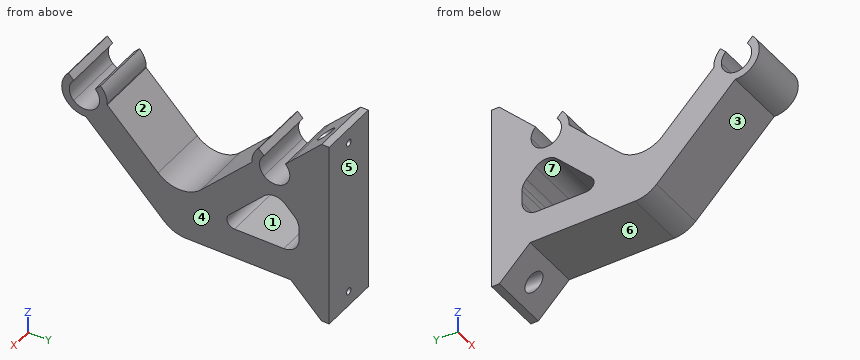
from build123d import *

# Parameters (mm, degrees)
F1_DEPTH = 50.8
F2_R     = 2.8575
F3_DEPTH = 224.1419342397
F5_R     = 6.35
F5_R_2   = 2.8575
F6_DEPTH = 217.7919342397


with BuildPart() as f1:
    # F0 (on Right) → F1 (new body)
    with BuildSketch(Plane.YZ):
        with BuildLine():
            Line((-66.2205500581, -66.2205500581), (-70.7106781187, -70.7106781187))
            ThreePointArc((-70.7106781187, -70.7106781187), (-65.8235712608, -75.2811893269), (-60.6417499855, -79.5146411593))
            ThreePointArc((-60.6417499855, -79.5146411593), (-62.1249501408, -72.3194552405), (-66.2205500581, -66.2205500581))
        make_face()
        with BuildLine():
            Line((-60.6704465476, -80.7509096897), (-70.7106781187, -70.7106781187))
            ThreePointArc((-70.7106781187, -70.7106781187), (-67.9576641768, -74.8308546487), (-66.9909342397, -79.6909342397))
            ThreePointArc((-66.9909342397, -79.6909342397), (-67.9576641768, -84.5510138308), (-70.7106781187, -88.6711903608))
            Line((-70.7106781187, -88.6711903608), (-66.2205500581, -93.1613184213))
            ThreePointArc((-66.2205500581, -93.1613184213), (-62.3007430389, -87.4680641731), (-60.6704465476, -80.7509096897))
        make_face()
        with BuildLine():
            ThreePointArc((-60.6417499855, -79.5146411593), (-65.8235712608, -75.2811893269), (-70.7106781187, -70.7106781187))
            Line((-70.7106781187, -70.7106781187), (-60.6704465476, -80.7509096897))
            ThreePointArc((-60.6704465476, -80.7509096897), (-60.648313746, -80.2211273486), (-60.6409342397, -79.6909342397))
            ThreePointArc((-60.6409342397, -79.6909342397), (-60.6411381773, -79.6027867559), (-60.6417499855, -79.5146411593))
        make_face()
        with BuildLine():
            Line((60.6704465476, -80.7509096897), (70.7106781187, -70.7106781187))
            ThreePointArc((70.7106781187, -70.7106781187), (65.8235712608, -75.2811893269), (60.6417499855, -79.5146411593))
            ThreePointArc((60.6417499855, -79.5146411593), (60.6460643138, -80.133008335), (60.6704465476, -80.7509096897))
        make_face()
        with BuildLine():
            ThreePointArc((60.6417499855, -79.5146411593), (65.8235712608, -75.2811893269), (70.7106781187, -70.7106781187))
            Line((70.7106781187, -70.7106781187), (66.2205500581, -66.2205500581))
            ThreePointArc((66.2205500581, -66.2205500581), (62.1249501408, -72.3194552405), (60.6417499855, -79.5146411593))
        make_face()
        with BuildLine():
            ThreePointArc((70.7106781187, -88.6711903608), (66.9909342397, -79.6909342397), (70.7106781187, -70.7106781187))
            Line((70.7106781187, -70.7106781187), (60.6704465476, -80.7509096897))
            ThreePointArc((60.6704465476, -80.7509096897), (62.3007430389, -87.4680641731), (66.2205500581, -93.1613184213))
            Line((66.2205500581, -93.1613184213), (70.7106781187, -88.6711903608))
        make_face()
        with BuildLine():
            ThreePointArc((98.7409342397, -79.6909342397), (97.2908393341, -72.4008148532), (93.1613184213, -66.2205500581))
            Line((93.1613184213, -66.2205500581), (88.6711903608, -70.7106781187))
            ThreePointArc((88.6711903608, -70.7106781187), (91.4242043026, -74.8308546487), (92.3909342397, -79.6909342397))
            ThreePointArc((92.3909342397, -79.6909342397), (91.4242043026, -84.5510138308), (88.6711903608, -88.6711903608))
            Line((88.6711903608, -88.6711903608), (93.1613184213, -93.1613184213))
            ThreePointArc((93.1613184213, -93.1613184213), (97.2908393341, -86.9810536263), (98.7409342397, -79.6909342397))
        make_face()
        Polygon((119.05, -40.3318684794), (93.1613184213, -66.2205500581), (125.4, -66.2205500581), (125.4, -40.3318684794), align=None)
        with BuildLine():
            Line((125.4, -66.2205500581), (93.1613184213, -66.2205500581))
            ThreePointArc((93.1613184213, -66.2205500581), (97.2908393341, -72.4008148532), (98.7409342397, -79.6909342397))
            ThreePointArc((98.7409342397, -79.6909342397), (97.2908393341, -86.9810536263), (93.1613184213, -93.1613184213))
            ThreePointArc((93.1613184213, -93.1613184213), (79.6909342397, -98.7409342397), (66.2205500581, -93.1613184213))
            Line((66.2205500581, -93.1613184213), (0, -159.3818684794))
            Line((0, -159.3818684794), (-66.2205500581, -93.1613184213))
            ThreePointArc((-66.2205500581, -93.1613184213), (-71.9138043064, -97.0811254405), (-78.6309587898, -98.7114219318))
            Line((-78.6309587898, -98.7114219318), (-12.7, -164.6423807216))
            ThreePointArc((-12.7, -164.6423807216), (-4.4596469399, -170.1484086052), (5.2605122421, -172.0818684794))
            Line((5.2605122421, -172.0818684794), (93.1613184213, -172.0818684794))
            Line((93.1613184213, -172.0818684794), (125.4, -172.0818684794))
            Line((125.4, -172.0818684794), (125.4, -119.1512092688))
            Line((125.4, -119.1512092688), (125.4, -66.2205500581))
        make_face()
        with BuildLine():
            ThreePointArc((96.2802561211, -114.2407683632), (98.0883415579, -116.5201524195), (99.3302370763, -119.1512092688))
            ThreePointArc((99.3302370763, -119.1512092688), (99.8314406767, -121.1587455105), (100, -123.2210244843))
            Line((100, -123.2210244843), (100, -133.9818684794))
            ThreePointArc((100, -133.9818684794), (96.2802561211, -142.9621246005), (87.3, -146.6818684794))
            Line((87.3, -146.6818684794), (45.9907683632, -146.6818684794))
            ThreePointArc((45.9907683632, -146.6818684794), (40.1241333318, -142.761908275), (41.5006403027, -135.8417404189))
            Line((41.5006403027, -135.8417404189), (70.7106781187, -106.6317026029))
            ThreePointArc((70.7106781187, -106.6317026029), (79.6909342397, -102.911958724), (88.6711903608, -106.6317026029))
            Line((88.6711903608, -106.6317026029), (96.2802561211, -114.2407683632))
        make_face(mode=Mode.SUBTRACT)
        with BuildLine():
            Line((-17.9605122421, -123.4608439952), (-60.6704465476, -80.7509096897))
            ThreePointArc((-60.6704465476, -80.7509096897), (-62.3007430389, -87.4680641731), (-66.2205500581, -93.1613184213))
            Line((-66.2205500581, -93.1613184213), (0, -159.3818684794))
            Line((0, -159.3818684794), (66.2205500581, -93.1613184213))
            ThreePointArc((66.2205500581, -93.1613184213), (62.3007430389, -87.4680641731), (60.6704465476, -80.7509096897))
            Line((60.6704465476, -80.7509096897), (17.9605122421, -123.4608439952))
            ThreePointArc((17.9605122421, -123.4608439952), (0, -130.900331753), (-17.9605122421, -123.4608439952))
        make_face()
        with BuildLine():
            Line((-88.6711903608, -70.7106781187), (-93.1613184213, -66.2205500581))
            ThreePointArc((-93.1613184213, -66.2205500581), (-97.0811254405, -87.4680641731), (-78.6309587898, -98.7114219318))
            Line((-78.6309587898, -98.7114219318), (-88.6711903608, -88.6711903608))
            ThreePointArc((-88.6711903608, -88.6711903608), (-92.3909342397, -79.6909342397), (-88.6711903608, -70.7106781187))
        make_face()
        with BuildLine():
            ThreePointArc((88.6711903608, -88.6711903608), (79.6909342397, -92.3909342397), (70.7106781187, -88.6711903608))
            Line((70.7106781187, -88.6711903608), (66.2205500581, -93.1613184213))
            ThreePointArc((66.2205500581, -93.1613184213), (79.6909342397, -98.7409342397), (93.1613184213, -93.1613184213))
            Line((93.1613184213, -93.1613184213), (88.6711903608, -88.6711903608))
        make_face()
        with BuildLine():
            Line((-66.2205500581, -93.1613184213), (-70.7106781187, -88.6711903608))
            ThreePointArc((-70.7106781187, -88.6711903608), (-79.6909342397, -92.3909342397), (-88.6711903608, -88.6711903608))
            Line((-88.6711903608, -88.6711903608), (-78.6309587898, -98.7114219318))
            ThreePointArc((-78.6309587898, -98.7114219318), (-71.9138043064, -97.0811254405), (-66.2205500581, -93.1613184213))
        make_face()
        Polygon((125.4, -197.9705500581), (125.4, -172.0818684794), (93.1613184213, -172.0818684794), (119.05, -197.9705500581), align=None)
    extrude(amount=F1_DEPTH)

    # F2 (on face) → F3 (cut, through all)
    with BuildSketch(Plane(origin=(0, 125.4, 0), x_dir=(-1, 0, 0), z_dir=(0, 1, 0))):
        with Locations((-25.4, -185.2705500581)):
            Circle(F2_R)
        with Locations((-25.4, -53.0318684794)):
            Circle(F2_R)
    extrude(amount=-F3_DEPTH, mode=Mode.SUBTRACT)

    # F5 (on offset) → F6 (cut, through all)
    with BuildSketch(Plane(origin=(0, 119.05, 0), x_dir=(-1, 0, 0), z_dir=(0, 1, 0))):
        with Locations((-25.4, -53.0318684794)):
            Circle(F5_R)
        with Locations((-25.4, -53.0318684794)):
            Circle(F5_R_2, mode=Mode.SUBTRACT)
        with Locations((-25.4, -185.2705500581)):
            Circle(F5_R)
        with Locations((-25.4, -185.2705500581)):
            Circle(F5_R_2, mode=Mode.SUBTRACT)
    extrude(amount=-F6_DEPTH, mode=Mode.SUBTRACT)


solid = f1.part
Can you work these out from the model? Positions are in its coordinate system, mm. Face numbers are marked on the shaded views. A direction names the side the tool comes from. Round coordinates to 2 decimals unless told otherwise and drop trailing zeros. Order: outer loops, then holes, each group sorted by start corner. A loop starts at its lowest first (then second) coordinate and runs counter-clockwise, first axis right, second up. Notation, with made-up numbers: M 2.5,89 L 35.5,89 A18 cw 35.5,117 Z; hole C -5,69.5 d4. An arc over 180 degrees is marked long. Use a Markdown table: item, result.
1) Imagine slicing it at B-B (x = 25.4). Give the number of separate pieces and of enclosed holes in the cut face, then the cut area to 3 significant figures.
Geometry says:
| item | result |
|---|---|
| separate pieces | 3 |
| enclosed holes | 1 |
| area | 11,700 mm² |
2) Imagine slicing it at A-A (y = 51). List the corners of the cut face in (x, z) for me.
Geometry says:
| item | result |
|---|---|
| outline | M 0,-172.08 L 50.8,-172.08 L 50.8,-146.68 L 0,-146.68 Z; M 0,-126.34 L 50.8,-126.34 L 50.8,-90.42 L 0,-90.42 Z |
3) Imagine slicing it at D-D (z = -110.5). List the corners of the cut face in (x, y) for me, then the cut area to 3 significant figures.
Geometry says:
| item | result |
|---|---|
| outline | M 0,-66.84 L 50.8,-66.84 L 50.8,-30.92 L 0,-30.92 Z; M 0,30.92 L 50.8,30.92 L 50.8,66.84 L 0,66.84 Z; M 0,92.54 L 50.8,92.54 L 50.8,125.4 L 0,125.4 Z |
| area | 5,320 mm² |
4) If I drill on line 1 along Y through (x, z) = (16, -80); line 2 along Z through (x, y) = (25.4, 123.5); line 3 along Y through (x, z) = (17.5, -104), over which ranges is the centre line in solid material (lowest first)?
Geometry says:
| item | result |
|---|---|
| line 1 | y = -98.74 to -92.39, -66.99 to -60.64, 60.64 to 66.99, 92.39 to 125.4 |
| line 2 | z = -197.97 to -188.13, -182.41 to -55.89, -50.17 to -40.33 |
| line 3 | y = -73.34 to -37.42, 37.42 to 74.55, 84.83 to 125.4 |
5) On a 3-axis mill with a long thin cutter (end or side, diameter ignored), from which of +Z, -Z, +X, -X, +Y, -Y can I reach the whole of each face in a straight line? I mean the marked faces 5, 6 and 7. Say none if no direction works.
Geometry says:
| item | result |
|---|---|
| face 5 | +Z, -Z, +X, -X, +Y |
| face 6 | -Z, +X, -X, -Y |
| face 7 | +X, -X |
6) I'm going to push flat-ended pins straight in: P1, Ø2, axis at x = 10, y = -47.5, coming from the -Z side; P2, Ø7.5, axis at x = 25.4, z = -53.03, coming from the -Y side; P3, Ø1.5, axis at x = 25, z = -134, coming from the -Y side; P4, Ø1, axis at y = 63.5, z = -116, coming from the -X side. Where does each tip first touch, or does it pass through?
Geometry says:
| item | result |
|---|---|
| P1 | stops at z = -130.84 |
| P2 | stops at y = 119.05 |
| P3 | stops at y = -44.09 |
| P4 | passes through |
7) If we mould it in two halves opening along Z, with no side actions, what happens to the marked faces 1, 2, 3 and 4? For each: +Z half, -Z half, draft (parallel to the pull), parting line (faces both ways), or undercut.
Geometry says:
| item | result |
|---|---|
| face 1 | undercut |
| face 2 | +Z half |
| face 3 | -Z half |
| face 4 | draft |
8) Imagine slicing it at C-C (z = -86). List the corners of the cut face in (x, y) for me.
Geometry says:
| item | result |
|---|---|
| outline | M 0,-97.67 L 50.8,-97.67 L 50.8,-90.71 L 0,-90.71 Z; M 0,-68.67 L 50.8,-68.67 L 50.8,-55.42 L 0,-55.42 Z; M 0,55.42 L 50.8,55.42 L 50.8,68.67 L 0,68.67 Z; M 0,90.71 L 50.8,90.71 L 50.8,125.4 L 0,125.4 Z |
